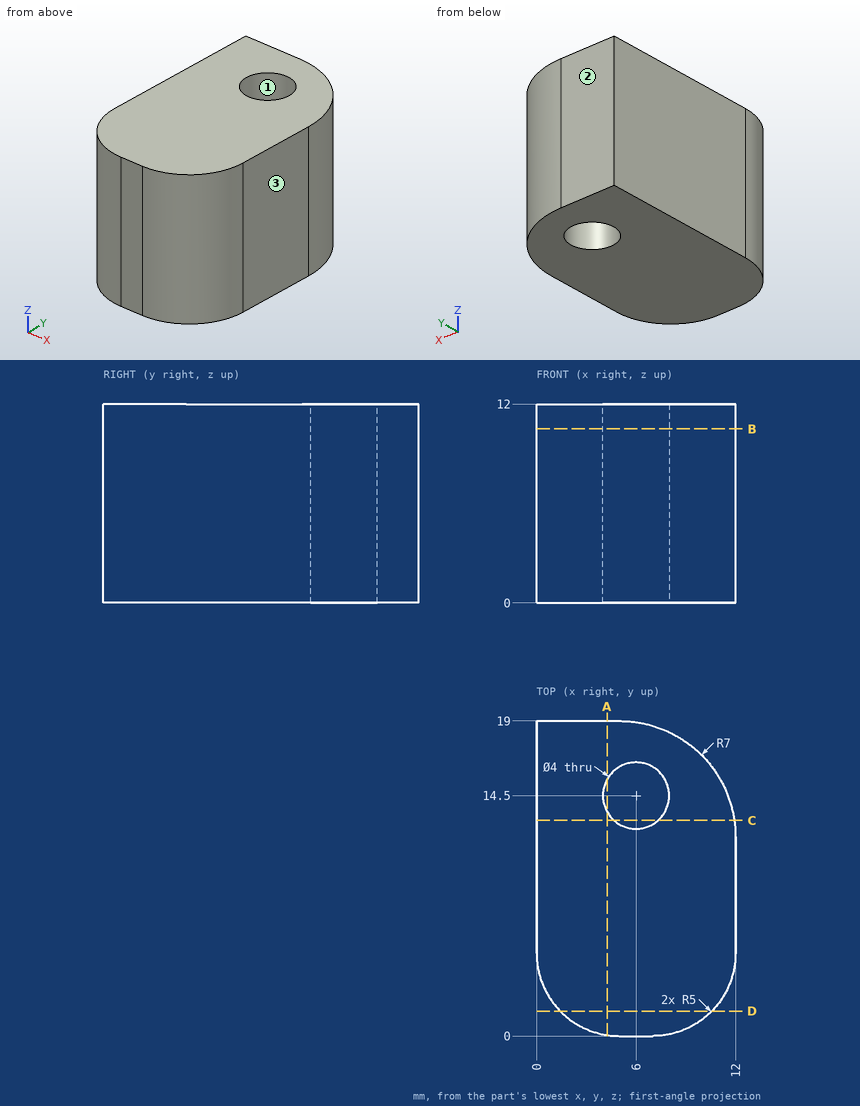
Print and shaded views of the part. All mm, measured from the part's lowest x, y and z. Give positions to 0.01 mm unless a question says otherwise; leave off trailing zeros. Loops run counter-clockwise (first coordinate to the right, second up) from the corner with the lowest first, then second, coordinate; pieces in that order, holes last.
1) Flat gauge pins, fed straight in: pin 1 Ø4 at (y, z) = (2, 4) entering from +X; pin 2 Ø5 at (x, y) = (6, 14.5) entering from -Z. Where does each tip first touch, or does it go through?
2) Pull direction X, two halves, no side cores. Call the marked faces 1, 2 and 3: +X half, -X half, draft (parallel to the pull), parting line (faces both ways), or undercut.
3) Wall check: line 1 (Y direction, x = 6, z = 5); line 2 (X direction, y = 17, z = 6.5); line 3 (X direction, y = 16, z = 9.75). Give the ranges that are in metal, low to high.
4) Saw through at C-C (y = 13). Write the cut outline in (x, z).
5) Saw through at B-B (z = 10.5). Write the cut outline in (x, y), plus the area to 3 significant figures.
6) Saw through at A-A (x = 4.25). Write the cut outline in (y, z).
7) Saw through at D-D (y = 1.5). Write the cut outline in (x, z), plus the area to 3 significant figures.
Answer block:
1. pin 1: stops at x = 11.9
1. pin 2: stops at z = 0
2. face 1: undercut
2. face 2: draft
2. face 3: +X half
3. line 1: y = 0 to 12.5, 16.5 to 18.93
3. line 2: x = 0 to 9.9
3. line 3: x = 0 to 4.68, 7.32 to 10.74
4. outline: (0, 0) - (4.68, 0) - (4.68, 12) - (0, 12) - close; (7.32, 0) - (11.93, 0) - (11.93, 12) - (7.32, 12) - close
5. outline: (0, 5) arc R5 ccw to (5, 0) - (7, 0) arc R5 ccw to (12, 5) - (12, 12) arc R7 ccw to (5, 19) - (0, 19) - close; hole circle Ø4 at (6, 14.5)
5. area: 194 mm2
6. outline: (0.06, 0) - (13.53, 0) - (13.53, 12) - (0.06, 12) - close; (15.47, 0) - (19, 0) - (19, 12) - (15.47, 12) - close
7. outline: (1.43, 0) - (10.57, 0) - (10.57, 12) - (1.43, 12) - close
7. area: 110 mm2
